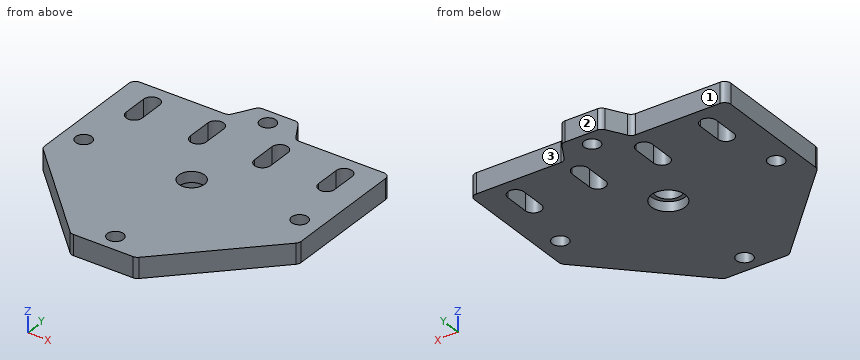
from build123d import *

# Parameters (mm, degrees)
SKETCH1_R                 = 4
SKETCH1_R_2               = 2.5
BOSS_EXTRUDE1_DEPTH       = 6.35
F_5_0MM_DOWEL_SLOT1_DEPTH = 6.35
SKETCH5_R                 = 5.25
CUT_EXTRUDE1_DEPTH        = 3


# Read off the part's stored shape, not the designer's step: Ø5.0mm Dowel Slot1
with BuildPart() as part:
    # Sketch1 → Boss-Extrude1 (new body)
    with BuildSketch(Plane.XY):
        with BuildLine():
            Line((-27.999999098, 10), (-1.639527193, 10))
            ThreePointArc((-1.639527193, 10), (-0.639527193, 10.267949192), (0.092523614, 11))
            Line((0.092523614, 11), (3.267950095, 16.5))
            ThreePointArc((3.267950095, 16.5), (4.000000902, 17.232050808), (5.000000902, 17.5))
            Line((5.000000902, 17.5), (15.000000902, 17.5))
            ThreePointArc((15.000000902, 17.5), (16.000000902, 17.232050808), (16.73205171, 16.5))
            Line((16.73205171, 16.5), (19.907478191, 11))
            ThreePointArc((19.907478191, 11), (20.639528998, 10.267949192), (21.639528998, 10))
            Line((21.639528998, 10), (48.000000902, 10))
            ThreePointArc((48.000000902, 10), (49.414214465, 9.414213562), (50.000000902, 8))
            Line((50.000000902, 8), (50.000000902, -29.321572875))
            ThreePointArc((50.000000902, -29.321572875), (49.847759967, -30.08693974), (49.414214465, -30.735786438))
            Line((49.414214465, -30.735786438), (20.73578734, -59.414213562))
            ThreePointArc((20.73578734, -59.414213562), (20.086940642, -59.847759065), (19.321573778, -60))
            Line((19.321573778, -60), (0.678428027, -60))
            ThreePointArc((0.678428027, -60), (-0.086938838, -59.847759065), (-0.735785535, -59.414213562))
            Line((-0.735785535, -59.414213562), (-29.41421266, -30.735786438))
            ThreePointArc((-29.41421266, -30.735786438), (-29.847758163, -30.08693974), (-29.999999098, -29.321572875))
            Line((-29.999999098, -29.321572875), (-29.999999098, 8))
            ThreePointArc((-29.999999098, 8), (-29.41421266, 9.414213562), (-27.999999098, 10))
        make_face()
        with Locations((10.000000902, -20.95)):
            Circle(SKETCH1_R, mode=Mode.SUBTRACT)
        with Locations((43.658284542, -20.95)):
            Circle(SKETCH1_R_2, mode=Mode.SUBTRACT)
        with Locations((10.000000902, -54.608282784)):
            Circle(SKETCH1_R_2, mode=Mode.SUBTRACT)
        with Locations((-23.658282737, -20.95)):
            Circle(SKETCH1_R_2, mode=Mode.SUBTRACT)
        with Locations(Location((10.000000902, 12.708282784, 0), (0, 0, 180))):
            Circle(SKETCH1_R_2, mode=Mode.SUBTRACT)
    extrude(amount=BOSS_EXTRUDE1_DEPTH)

    # Ø5.0mm Dowel Slot1 outline → Ø5.0mm Dowel Slot1 (cut)
    with BuildSketch(Plane.XY):
        with BuildLine():
            Line((22.5, -3.85), (22.5, 3.85))
            ThreePointArc((22.5, 3.85), (20, 6.35), (17.5, 3.85))
            Line((17.5, 3.85), (17.5, -3.85))
            ThreePointArc((17.5, -3.85), (20, -6.35), (22.5, -3.85))
        make_face()
        with BuildLine():
            Line((-17.5, -3.85), (-17.5, 3.85))
            ThreePointArc((-17.5, 3.85), (-20, 6.35), (-22.5, 3.85))
            Line((-22.5, 3.85), (-22.5, -3.85))
            ThreePointArc((-22.5, -3.85), (-20, -6.35), (-17.5, -3.85))
        make_face()
        with BuildLine():
            Line((2.5, -3.85), (2.5, 3.85))
            ThreePointArc((2.5, 3.85), (0, 6.35), (-2.5, 3.85))
            Line((-2.5, 3.85), (-2.5, -3.85))
            ThreePointArc((-2.5, -3.85), (0, -6.35), (2.5, -3.85))
        make_face()
        with BuildLine():
            Line((42.5, -3.85), (42.5, 3.85))
            ThreePointArc((42.5, 3.85), (40, 6.35), (37.5, 3.85))
            Line((37.5, 3.85), (37.5, -3.85))
            ThreePointArc((37.5, -3.85), (40, -6.35), (42.5, -3.85))
        make_face()
    extrude(amount=F_5_0MM_DOWEL_SLOT1_DEPTH, mode=Mode.SUBTRACT)

    # Sketch5 → Cut-Extrude1 (cut)
    with BuildSketch(Plane(origin=(0, 0, 0), x_dir=(-1, 0, 0), z_dir=(0, 0, -1))):
        with Locations((-10.000000902, -20.95)):
            Circle(SKETCH5_R)
    extrude(amount=-CUT_EXTRUDE1_DEPTH, mode=Mode.SUBTRACT)


solid = part.part
Build history of the part. All positions in model axes, mm. Face numbers are marked on the shaded views. A direction names the side the tool comes from. Coordinates: 2 decimals unless noted, no trailing zeros. Write each loop counter-clockwise with the first axis right and the second up, starting at its lowest first coordinate (ties: lowest second). Pieces come first, ordered by that corner, then holes. Notation, with made-up numbers: (69, 11) -> (124, 11) arc R18 cw to (124, 17) -> close; hole circle Ø4 at (46.5, 46). An arc over 180 degrees is marked (long way). Use CSV: the item, a comma, the result in double quotes. Start each with the question number.
Q1. Cut at C-C, the plane x = 10. List the corners of the cut face in (y, z).
Q2. Drill centre lines: probe 1 along X at (y, z) = (0.5, 5.75); probe 2 along Y at (x, z) = (10, 3.5); probe 3 along Y at (x, z) = (10, 2.75). Where is each one in solid material? Low to high.
Q3. 3-axis set-ups, long thin cutter, end or side, ignore diameter. For the marked faces 1, 2 and 3: which of +Z, -Z, +X, -X, +Y, -Y reach the whole face in a straight line?
Q4. Flat gauge pins, fed straight in: pin 1 Ø4 at (x, y) = (10, -54.61) entering from -Z; pin 2 Ø1.9 at (x, z) = (39.5, 1.5) entering from +Y; pin 3 Ø1 at (x, z) = (-17.5, 3.5) entering from -Y. Where does each tip first touch, or does it go through?
Q5. Cut at D-D, the plane x = -20. List the corners of the cut face in (y, z).
Q6. Cut at B-B, the plane y = -20.95. List the corners of the cut face in (x, z), then the cut area to 3 significant figures.
Q7. Cut at A-A, the plane y = 0.5. List the corners of the cut face in (x, z), then the cut area to 3 significant figures.
Checked values:
1,outline,"(-60, 0) -> (-57.11, 0) -> (-57.11, 6.35) -> (-60, 6.35) -> close; (-52.11, 0) -> (-26.2, 0) -> (-26.2, 3) -> (-24.95, 3) -> (-24.95, 6.35) -> (-52.11, 6.35) -> close; (-16.95, 3) -> (-15.7, 3) -> (-15.7, 0) -> (10.21, 0) -> (10.21, 6.35) -> (-16.95, 6.35) -> close; (15.21, 0) -> (17.5, 0) -> (17.5, 6.35) -> (15.21, 6.35) -> close"
2,probe 1,"x = -30 to -22.5, -17.5 to -2.5, 2.5 to 17.5, 22.5 to 37.5, 42.5 to 50"
2,probe 2,"y = -60 to -57.11, -52.11 to -24.95, -16.95 to 10.21, 15.21 to 17.5"
2,probe 3,"y = -60 to -57.11, -52.11 to -26.2, -15.7 to 10.21, 15.21 to 17.5"
3,face 1,"+Z, -Z, -X, +Y"
3,face 2,"+Z, -Z, +X, -X, +Y"
3,face 3,"+Z, -Z, +X, +Y"
4,pin 1,"passes through"
4,pin 2,"stops at y = 10"
4,pin 3,"stops at y = -43.15"
5,outline,"(-40.15, 0) -> (-6.35, 0) -> (-6.35, 6.35) -> (-40.15, 6.35) -> close; (6.35, 0) -> (10, 0) -> (10, 6.35) -> (6.35, 6.35) -> close"
6,outline,"(-30, 0) -> (-26.16, 0) -> (-26.16, 6.35) -> (-30, 6.35) -> close; (-21.16, 0) -> (4.75, 0) -> (4.75, 3) -> (6, 3) -> (6, 6.35) -> (-21.16, 6.35) -> close; (14, 3) -> (15.25, 3) -> (15.25, 0) -> (41.16, 0) -> (41.16, 6.35) -> (14, 6.35) -> close; (46.16, 0) -> (50, 0) -> (50, 6.35) -> (46.16, 6.35) -> close"
6,area,"386 mm²"
7,outline,"(-30, 0) -> (-22.5, 0) -> (-22.5, 6.35) -> (-30, 6.35) -> close; (-17.5, 0) -> (-2.5, 0) -> (-2.5, 6.35) -> (-17.5, 6.35) -> close; (2.5, 0) -> (17.5, 0) -> (17.5, 6.35) -> (2.5, 6.35) -> close; (22.5, 0) -> (37.5, 0) -> (37.5, 6.35) -> (22.5, 6.35) -> close; (42.5, 0) -> (50, 0) -> (50, 6.35) -> (42.5, 6.35) -> close"
7,area,"381 mm²"
